Source: CAD feature listing. Evaluate the final solid. Frame: model axes, mm. Face numbers are marked on the shaded views. A direction names the side the tool comes from. Give positions to 0.01 mm unless a question says otherwise; leave off trailing zeros. Order: outer loops, then holes, each group sorted by start corner. A loop starts at its lowest first (then second) coordinate and runs counter-clockwise, first axis right, second up. Notation, with made-up numbers: M 43,12 L 100,12 A27 ccw 100,44 Z; hole C -24,48 d10. An arc over 180 degrees is marked long. Return JSON: item names as keys, results as strings.
from build123d import *

# Parameters (mm, degrees)
F1_DEPTH = 5
F2_W     = 10.7573593129
F2_H     = 2
F3_DEPTH = 3
F4_W     = 10.7573593129
F4_H     = 2
F5_DEPTH = 3
F6_W     = 3
F6_H     = 2
F7_DEPTH = 1
F8_W     = 1.5857864376
F8_H     = 2
F9_DEPTH = 1.4
F10_R    = 2


with BuildPart() as f1:
    # F0 (on Top) → F1 (new body)
    with BuildSketch(Plane.XY):
        Polygon((-11.313708499, 5.6568542495), (-1.6568542495, -4), (12, -4), (12, 3), (1.2426406871, 3), (-6.3639610307, 10.6066017178), align=None)
    extrude(amount=F1_DEPTH)

    # F2 (on face) → F3 (cut)
    with BuildSketch(Plane(origin=(2.1213203436, 2.1213203436, 0), x_dir=(-0.7071067812, 0.7071067812, 0), z_dir=(0.7071067812, 0.7071067812, 0))):
        with Locations((6.6213203436, 2.5)):
            Rectangle(F2_W, F2_H)
    extrude(amount=-F3_DEPTH, mode=Mode.SUBTRACT)

    # F4 (on face) → F5 (cut)
    with BuildSketch(Plane(origin=(0, 3, 0), x_dir=(-1, 0, 0), z_dir=(0, 1, 0))):
        with Locations((-6.6213203436, 2.5)):
            Rectangle(F4_W, F4_H)
    extrude(amount=-F5_DEPTH, mode=Mode.SUBTRACT)

    # F6 (on face) → F7 (cut)
    with BuildSketch(Plane.YZ.offset(1.2426406871)):
        with Locations((1.5, 2.5)):
            Rectangle(F6_W, F6_H)
    extrude(amount=-F7_DEPTH, mode=Mode.SUBTRACT)

    # F8 (on face) → F9 (cut)
    with BuildSketch(Plane(origin=(-0.8786796564, 0.8786796564, 0), x_dir=(-0.7071067812, -0.7071067812, 0), z_dir=(-0.7071067812, 0.7071067812, 0))):
        with Locations((-0.7928932188, 2.5)):
            Rectangle(F8_W, F8_H)
    extrude(amount=-F9_DEPTH, mode=Mode.SUBTRACT)

    # F10
    f10_edges = [f1.edges().sort_by_distance(p)[0] for p in [
        (-1.656854, -4, 2.5),
        (-11.313708, 5.656854, 2.5),
        (12, -4, 2.5),
        (12, 3, 4.25),
        (12, 3, 0.75),
        (-6.363961, 10.606602, 4.25),
        (-6.363961, 10.606602, 0.75),
    ]]
    fillet(f10_edges, radius=F10_R)


solid = f1.part
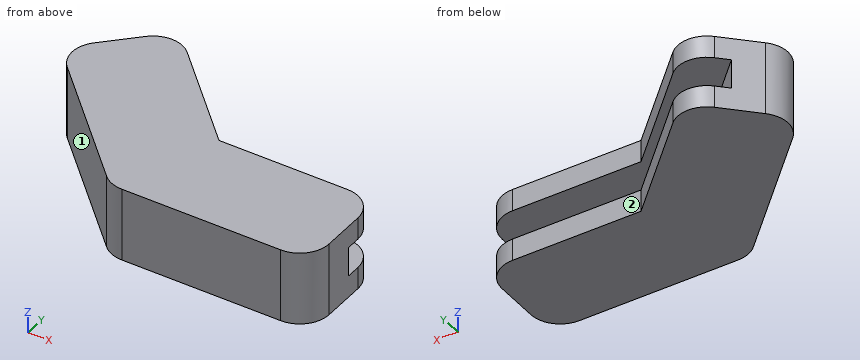
1. First-contact query: pin 1 (1.2 mm diameter, centred on x = 3.5, z = 1, fed in from +Y); pin 2 (1 mm diameter, centred on y = 3.5, z = 2.5, fed in from -X); pin 3 (4 mm diameter, centred on x = 6, y = 6.5, fed in from -Z); pin 4 (1 mm diameter, centred on x = 3.5, z = 2.5, fed in from +Y). Flat tips, straight axial feed; report the tip coordinate or a pass-through.
Evaluation:
{"pin 1": "stops at y = 3", "pin 2": "stops at x = -9.66", "pin 3": "passes through", "pin 4": "stops at y = 0"}
2. Section query A-A (x = 8). Return loops of the section in (y, z).
Evaluation:
{"outline": "M -4,0 L 3,0 L 3,1.5 L 0,1.5 L 0,3.5 L 3,3.5 L 3,5 L -4,5 Z"}
3. Ray query, probe 1 along Z at (x, y) = (9.25, 0.5); probe 2 along Y at (x, z) = (10, 0.5); probe 3 along Y at (x, z) = (0, 4.15). Return the intervals inside material, ascending.
Evaluation:
{"probe 1": "z = 0 to 1.5, 3.5 to 5", "probe 2": "y = -4 to 3", "probe 3": "y = -4 to 4.24"}
4. Section query D-D (z = 0.4). Return loops of the section in (x, y).
Evaluation:
{"outline": "M -9.9,4.24 L -2.24,-3.41 A2 ccw -0.83,-4 L 10,-4 A2 ccw 12,-2 L 12,1 A2 ccw 10,3 L 1.24,3 L -4.95,9.19 A2 ccw -7.78,9.19 L -9.9,7.07 A2 ccw Z"}
5. Section query C-C (y = 5.25). Return loops of the section in (x, z).
Evaluation:
{"outline": "M -10.44,0 L -1.01,0 L -1.01,1.5 L -5.25,1.5 L -5.25,3.5 L -1.01,3.5 L -1.01,5 L -10.44,5 Z"}
6. Set-up query: the marked faces 1 and 2. Return all of +Z, -Z, +X, -X, +Y, -Y with unobstructed straight access to the full face (end or side cutting, diameter ignored); none if empty.
Evaluation:
{"face 1": "+Z, -Z, -X, -Y", "face 2": "+Z, -Z, +X, +Y"}
